The model under review builds one solid part; all positions refer to its coordinate system, in mm. A direction names the side the tool comes from. Round coordinates to 2 decimals unless told otherwise and drop trailing zeros. Order: outer loops, then holes, each group sorted by start corner. A loop starts at its lowest first (then second) coordinate and runs counter-clockwise, first axis right, second up. Notation, with made-up numbers: (46.5, 69) -> (81.5, 69) arc R15 cw to (81.5, 97) -> close; hole circle Ø1 at (20.5, 27). An arc over 180 degrees is marked (long way). Use a Markdown table: item, result. Add a question column.
```python
from build123d import *

# Parameters (mm, degrees)
SKETCH1_R           = 2.5
SKETCH1_R_2         = 0.75
BOSS_EXTRUDE1_DEPTH = 2.25
SKETCH2_R           = 3.879501895
SKETCH2_R_2         = 2.5
BOSS_EXTRUDE2_DEPTH = 2.25
SKETCH3_R           = 2.5
SKETCH3_R_2         = 2.008527967
BOSS_EXTRUDE3_DEPTH = 1
SKETCH4_R           = 3.8
SKETCH4_R_2         = 3
CUT_EXTRUDE1_DEPTH  = 0.5


with BuildPart() as part:
    # Sketch1 → Boss-Extrude1 (new body)
    with BuildSketch(Plane(origin=(0, 0, 0), x_dir=(1, 0, 0), z_dir=(0, 1, 0))):
        with BuildLine():
            Line((-1.6, 19), (-3.75, 3.885550154))
            ThreePointArc((-3.75, 3.885550154), (-5.4, 0), (-3.75, -3.885550154))
            Line((-3.75, -3.885550154), (-1.6, -19))
            ThreePointArc((-1.6, -19), (0, -20.6), (1.6, -19))
            Line((1.6, -19), (3.75, -3.885550154))
            ThreePointArc((3.75, -3.885550154), (5.4, 0), (3.75, 3.885550154))
            Line((3.75, 3.885550154), (1.6, 19))
            ThreePointArc((1.6, 19), (0, 20.6), (-1.6, 19))
        make_face()
        Circle(SKETCH1_R, mode=Mode.SUBTRACT)
        with Locations((0, -19)):
            Circle(SKETCH1_R_2, mode=Mode.SUBTRACT)
        with Locations((0, 19)):
            Circle(SKETCH1_R_2, mode=Mode.SUBTRACT)
        with Locations((0, 15.5)):
            Circle(SKETCH1_R_2, mode=Mode.SUBTRACT)
        with Locations((0, 12)):
            Circle(SKETCH1_R_2, mode=Mode.SUBTRACT)
        with Locations((0, 8.5)):
            Circle(SKETCH1_R_2, mode=Mode.SUBTRACT)
        with Locations((0, -15.5)):
            Circle(SKETCH1_R_2, mode=Mode.SUBTRACT)
        with Locations((0, -12)):
            Circle(SKETCH1_R_2, mode=Mode.SUBTRACT)
        with Locations((0, -8.5)):
            Circle(SKETCH1_R_2, mode=Mode.SUBTRACT)
    extrude(amount=BOSS_EXTRUDE1_DEPTH)

    # Sketch2 → Boss-Extrude2 (add)
    with BuildSketch(Plane(origin=(0, 2.25, 0), x_dir=(1, 0, 0), z_dir=(0, 1, 0))):
        Circle(SKETCH2_R)
        Circle(SKETCH2_R_2, mode=Mode.SUBTRACT)
    extrude(amount=BOSS_EXTRUDE2_DEPTH)

    # Sketch3 → Boss-Extrude3 (add)
    with BuildSketch(Plane.XZ):
        Circle(SKETCH3_R)
        Circle(SKETCH3_R_2, mode=Mode.SUBTRACT)
    extrude(amount=-BOSS_EXTRUDE3_DEPTH)

    # Sketch4 → Cut-Extrude1 (cut)
    with BuildSketch(Plane.XZ):
        Circle(SKETCH4_R)
        Circle(SKETCH4_R_2, mode=Mode.SUBTRACT)
    extrude(amount=-CUT_EXTRUDE1_DEPTH, mode=Mode.SUBTRACT)


solid = part.part
```
Q1. Add section C-C, the plane y = 3.95. Give the boundary of the cut face in (x, z).
Q2. To check wall thickness, follow line 1 along Y through (x, z) = (-3.75, 2.5); line 2 along X through (y, z) = (2, 11.5); line 3 along X through (y, z) = (1.5, -8). State the ranges of each line that lie inside material, in increasing order.
Q3. Add section D-D, the plane z = 15.5. Give the boundary of the cut face in (x, y), then the cut area to 3 significant figures.
Q4. Add section B-B, the plane z = -0.5. Give the boundary of the cut face in (x, y).
Q5. Add section A-A, the plane x = 1.25. Give the boundary of the cut face in (y, z).
Q6. For faces 1 (the face through (-0.54, 2.73, 2.44)), 2 (the face through (-0.163, 1.109, -18.268)), 3 (the face through (3, 0.5, 1)), list the 3-axis set-ups (+Z, -Z, +X, -X, +Y, -Y) from which the entire face can be reached by the end or side of a thin tool; tool diameter is ignored.
Q7. For pin 1 (1.5 mm diameter, centred on y = 0.5, z = 13.5, fed in from -X); pin 2 (2 mm diameter, centred on y = 0.5, z = 12, fed in from -X); pin 3 (1.5 mm diameter, centred on y = 2, z = -7, fed in from -X), all flat-tipped, find the tip position at first contact; note any pin that passes through.
Q8. Draft analysis for pull direction X (two halves, no side actions). For faces 4 (the face through (-0.841, 3.359, 3.787)), 5 (the face through (-3, 0.2, 0.1)), 6 (the face through (1, 0, -2)), state which applies: released by +X, released by -X, zero draft, split by the parting line, or undercut.
Return value:
| question | item | result |
|---|---|---|
| 1 | outline | circle Ø7.76 at (0, 0); hole circle Ø5 at (0, 0) |
| 2 | line 1 | 0 to 2.25 |
| 2 | line 2 | -2.67 to -0.56, 0.56 to 2.67 |
| 2 | line 3 | -3.16 to -0.56, 0.56 to 3.16 |
| 3 | outline | (-2.1, 0) -> (-0.75, 0) -> (-0.75, 2.25) -> (-2.1, 2.25) -> close; (0.75, 0) -> (2.1, 0) -> (2.1, 2.25) -> (0.75, 2.25) -> close |
| 3 | area | 6.07 mm² |
| 4 | outline | (-5.38, 0) -> (-3.77, 0) -> (-3.77, 0.5) -> (-2.96, 0.5) -> (-2.96, 0) -> (-1.95, 0) -> (-1.95, 1) -> (-2.45, 1) -> (-2.45, 4.5) -> (-3.85, 4.5) -> (-3.85, 2.25) -> (-5.38, 2.25) -> close; (1.95, 0) -> (2.96, 0) -> (2.96, 0.5) -> (3.77, 0.5) -> (3.77, 0) -> (5.38, 0) -> (5.38, 2.25) -> (3.85, 2.25) -> (3.85, 4.5) -> (2.45, 4.5) -> (2.45, 1) -> (1.95, 1) -> close |
| 5 | outline | (0, -20) -> (2.25, -20) -> (2.25, -3.67) -> (4.5, -3.67) -> (4.5, -2.17) -> (1, -2.17) -> (1, -1.57) -> (0, -1.57) -> (0, -2.73) -> (0.5, -2.73) -> (0.5, -3.59) -> (0, -3.59) -> close; (0, 1.57) -> (1, 1.57) -> (1, 2.17) -> (4.5, 2.17) -> (4.5, 3.67) -> (2.25, 3.67) -> (2.25, 20) -> (0, 20) -> (0, 3.59) -> (0.5, 3.59) -> (0.5, 2.73) -> (0, 2.73) -> close |
| 6 | face 1 | +Y |
| 6 | face 2 | +Y, -Y |
| 6 | face 3 | -Y |
| 7 | pin 1 | x = -2.49 |
| 7 | pin 2 | x = -2.74 |
| 7 | pin 3 | x = -3.41 |
| 8 | face 4 | split by the parting line |
| 8 | face 5 | undercut |
| 8 | face 6 | zero draft |
